from build123d import *

# Parameters (mm, degrees)
F1_DEPTH = 50.8
F2_DEPTH = 2.54
F5_START = 43.18
F5_DEPTH = 1.016
F6_START = -61.722
F4_W     = 5.842
F4_H     = 12.7
F4_W_2   = 3.81
F4_H_2   = 38.1
F6_DEPTH = 1.524


# Not quite as in the source:
# - a feature of the source that left no trace in its solid (it failed there, or was rolled back) is left out


with BuildPart() as f1:
    # F0 (on Right) → F1 (new body)
    with BuildSketch(Plane.YZ):
        Polygon((-61.698825866, 55.9749106665), (-61.698825866, -45.4361034706), (65.301174134, -45.5878325482), (65.301174134, -27.8078325482), (62.494367, -23.5736580464), (62.494367, 41.5807361647), (65.301174134, 45.8149106665), (65.301174134, 55.9749106665), align=None)
        Polygon((-55.3488239149, -39.093683444), (-55.3488239149, 49.6249087155), (58.951172183, 49.6249087155), (58.951172183, -39.2302396091), align=None, mode=Mode.SUBTRACT)
        with BuildLine():
            Line((65.301174134, -45.5878325482), (-61.698825866, -45.4361034706))
            add(Edge.make_bspline(
                [(-65.5058175325, -55.8386668563), (-64.7629052579, -54.5340589091), (-63.1453130575, -51.6934494428), (-62.2064804259, -47.6321617795), (-61.698825866, -45.4361034706)],
                knots=[0, 0, 0, 0, 0.4592704357, 1, 1, 1, 1], degree=3))
            Line((-65.5058175325, -55.8386668563), (68.9185634255, -55.8386668563))
            add(Edge.make_bspline(
                [(68.9185634255, -55.8386668563), (67.8020531364, -54.0848642317), (65.6584922314, -50.7307193347), (65.4183999928, -47.2370915893), (65.301174134, -45.5878325482)],
                knots=[0, 0, 0, 0, 0.5226245331, 1, 1, 1, 1], degree=3))
        make_face()
    extrude(amount=F1_DEPTH)

    # F0 (on Right) → F2 (join)
    with BuildSketch(Plane.YZ):
        Polygon((58.951172183, 49.6249087155), (-55.3488239149, 49.6249087155), (-55.3488239149, -39.093683444), (58.951172183, -39.2302396091), align=None)
    extrude(amount=F2_DEPTH)

    # F2_face (on face) → F5 (join)
    with BuildSketch(Plane(origin=(2.54, 1.8158237937, 5.2314648434), x_dir=(0, 1, 0), z_dir=(1, 0, 0)).offset(F5_START)):
        Polygon((57.1353483893, -44.4617044525), (57.1353483893, 44.3934438721), (-57.1646477086, 44.3934438721), (-57.1646477086, -44.3251482873), align=None)
    extrude(amount=F5_DEPTH)

    # F4 (on Front) → F6 (join)
    with BuildSketch(Plane.XZ.offset(F6_START)):
        with BuildLine():
            Line((39.7206060588, -9.1834223449), (39.7206060588, 28.9165776551))
            Line((39.7206060588, 28.9165776551), (33.9717225262, 28.9165776551))
            ThreePointArc((33.9717225262, 28.9165776551), (31.8466060588, 27.6465776551), (29.7214895914, 28.9165776551))
            Line((29.7214895914, 28.9165776551), (22.506811127, 28.9165776551))
            ThreePointArc((22.506811127, 28.9165776551), (20.3816946596, 27.6465776551), (18.2565781922, 28.9165776551))
            Line((18.2565781922, 28.9165776551), (11.7806060588, 28.9165776551))
            Line((11.7806060588, 28.9165776551), (11.7806060588, -9.1834223449))
            Line((11.7806060588, -9.1834223449), (39.7206060588, -9.1834223449))
        make_face()
        with Locations((19.1466060588, 0.9765776551)):
            Rectangle(F4_W, F4_H, mode=Mode.SUBTRACT)
        with Locations((32.3546060588, 0.9765776551)):
            Rectangle(F4_W, F4_H, mode=Mode.SUBTRACT)
        with Locations((19.1466060588, 18.1998224765)):
            Rectangle(F4_W, F4_H, mode=Mode.SUBTRACT)
        with Locations((32.3546060588, 18.2028314263)):
            Rectangle(F4_W, F4_H, mode=Mode.SUBTRACT)
        with BuildLine():
            Line((33.9717225262, 28.9165776551), (39.7206060588, 28.9165776551))
            ThreePointArc((39.7206060588, 28.9165776551), (38.6315341138, 32.4725776551), (35.7378860588, 34.8088170767))
            Line((35.7378860588, 34.8088170767), (15.7633260588, 34.8088170767))
            ThreePointArc((15.7633260588, 34.8088170767), (12.8696780038, 32.4725776551), (11.7806060588, 28.9165776551))
            Line((11.7806060588, 28.9165776551), (18.2565781922, 28.9165776551))
            ThreePointArc((18.2565781922, 28.9165776551), (19.7923463058, 32.3995002004), (22.7946946596, 30.0595776551))
            ThreePointArc((22.7946946596, 30.0595776551), (22.7216172049, 29.4702293013), (22.506811127, 28.9165776551))
            Line((22.506811127, 28.9165776551), (29.7214895914, 28.9165776551))
            ThreePointArc((29.7214895914, 28.9165776551), (31.2572577051, 32.3995002004), (34.2596060588, 30.0595776551))
            ThreePointArc((34.2596060588, 30.0595776551), (34.1865286041, 29.4702293013), (33.9717225262, 28.9165776551))
        make_face()
        with Locations((7.3356060588, 9.8665776551)):
            Rectangle(F4_W_2, F4_H_2)
    extrude(amount=-F6_DEPTH)


solid = f1.part
Geometry check sheet. Reference: the model listing, model coordinates, mm. A direction names the side the tool comes from. Round coordinates to 2 decimals unless told otherwise and drop trailing zeros. Write each loop counter-clockwise with the first axis right and the second up, starting at its lowest first coordinate (ties: lowest second). Pieces come first, ordered by that corner, then holes.
Item 1: Section check A-A (z = -12.5). Record the boundary of the cut face in (x, y), plus the area to 3 significant figures.
Determined:
outline: (0, -61.7) - (50.8, -61.7) - (50.8, -55.35) - (46.74, -55.35) - (46.74, 58.95) - (50.8, 58.95) - (50.8, 62.49) - (0, 62.49) - close; hole (2.54, -55.35) - (45.72, -55.35) - (45.72, 58.95) - (2.54, 58.95) - close
area: 909 mm2
Item 2: Access from +Z, -Z, +X, -X, +Y, -Y to the whole of each face (thin tool, end or side, straight path). Record for faces 1 (the face through (26, 63.246, 13)), 2 (the face through (25, 65.301, 51)), 3 (the face through (20, 62.494, 30)).
Determined:
face 1: +X, -X, +Y
face 2: +Z, +X, -X, +Y
face 3: +Y
Item 3: Go/stop test with flat-tipped pins: pin 1 Ø6.5 at (x, z) = (18.5, 0) entering from +Y; pin 2 Ø14 at (x, z) = (28, -39.5) entering from +Y; pin 3 Ø5 at (x, z) = (8.5, -18.5) entering from -Y. Record where each tip stops, or that it passes through.
Determined:
pin 1: stops at y = 63.25
pin 2: stops at y = 65.37
pin 3: stops at y = -61.7
Item 4: Section check B-B (y = 22). Record the boundary of the cut face in (x, z).
Determined:
outline: (0, -55.84) - (50.8, -55.84) - (50.8, -39.19) - (46.74, -39.19) - (46.74, 49.62) - (50.8, 49.62) - (50.8, 55.97) - (0, 55.97) - close; hole (2.54, -39.19) - (45.72, -39.19) - (45.72, 49.62) - (2.54, 49.62) - close
Item 5: Material ranges on line 1 along X through (y, z) = (55, -20); line 2 along Y through (x, z) = (15, 21.5); line 3 along Y through (x, z) = (10, -35.5), recorded low to high.
Determined:
line 1: x = 0 to 2.54, 45.72 to 46.74
line 2: y = -61.7 to -55.35, 58.95 to 63.25
line 3: y = -61.7 to -55.35, 58.95 to 65.3
Item 6: Mould release check, pull along X, two halves, no side actions. Record for faces 4 (the face through (19, 62.494, 18)), 5 (the face through (25, 65.301, -37)), 6 (the face through (12.9, 62.86, 32.52)): +X half, -X half, draft (parallel to the pull), parting line (faces both ways), or undercut.
Determined:
face 4: undercut
face 5: draft
face 6: -X half
